from build123d import *

# Parameters (mm, degrees)
SKETCH1_R                        = 12.000000003
SKETCH1_R_2                      = 8.500000018
BOSS_EXTRUDE1_DEPTH              = 4.7625
SKETCH1_4_R                      = 9.525
CUT_EXTRUDE1_DEPTH               = 1.5875
F_10_32_TAPPED_HOLE1_D           = 4.0386
BOSS_EXTRUDE3_START              = -0.79375
SKETCH7_R                        = 8.500000018
SKETCH7_R_2                      = 6.5
BOSS_EXTRUDE3_DEPTH              = 0.79375
F_17_64_0_26563_DIAMETER_HOLE1_D = 6.747002
CUT_EXTRUDE2_DEPTH               = 0.7366


with BuildPart() as part:
    # Sketch1 → Boss-Extrude1 (new body)
    with BuildSketch(Plane.XY):
        with BuildLine():
            Line((-70.300649756, 35.543758941), (-22.715793489, -19.601472909))
            ThreePointArc((-22.715793489, -19.601472909), (6.372007721, -29.319320109), (28.80246523, -8.404939663))
            Line((28.80246523, -8.404939663), (49.20643424, 61.516396068))
            ThreePointArc((49.20643424, 61.516396068), (48.977980792, 61.993965606), (48.478121662, 61.819596767))
            ThreePointArc((48.478121662, 61.819596767), (47.697638407, 60.484610946), (46.853975269, 59.18862724))
            ThreePointArc((46.853975269, 59.18862724), (46.782773661, 59.083463588), (46.711157924, 58.978581516))
            ThreePointArc((46.711157924, 58.978581516), (13.35804262, 45.469068231), (-11.695774538, 71.300125033))
            ThreePointArc((-11.695774538, 71.300125033), (-16.142405131, 74.275551921), (-18.952954781, 69.722915382))
            ThreePointArc((-18.952954781, 69.722915382), (-31.025391021, 35.82315688), (-66.977119299, 34.270553581))
            ThreePointArc((-66.977119299, 34.270553581), (-67.0858071, 34.336250039), (-67.194235, 34.402374566))
            ThreePointArc((-67.194235, 34.402374566), (-68.499704148, 35.231284429), (-69.763880718, 36.121901549))
            ThreePointArc((-69.763880718, 36.121901549), (-70.291023197, 36.073070731), (-70.300649756, 35.543758941))
        make_face()
        Circle(SKETCH1_R, mode=Mode.SUBTRACT)
        with Locations((-7.832512348, 36.039494433)):
            Circle(SKETCH1_R_2, mode=Mode.SUBTRACT)
    extrude(amount=-BOSS_EXTRUDE1_DEPTH)

    # Sketch1_4 → Cut-Extrude1 (cut)
    with BuildSketch(Plane.XY):
        with Locations((-36.319050549, 15.602840887)):
            Circle(SKETCH1_4_R)
        with Locations((26.566795152, 29.269907275)):
            Circle(SKETCH1_4_R)
    extrude(amount=-CUT_EXTRUDE1_DEPTH, mode=Mode.SUBTRACT)

    # 10-32 Tapped Hole1 (through all)
    with Locations(Plane.XY):
        with Locations((-15.353270713, 70.644524994)):
            Hole(F_10_32_TAPPED_HOLE1_D / 2)

    # Sketch7 → Boss-Extrude3 (add)
    with BuildSketch(Plane(origin=(0, 0, -4.7625), x_dir=(-1, 0, 0), z_dir=(0, 0, -1)).offset(BOSS_EXTRUDE3_START)):
        with Locations(Location((7.832512348, 36.039494433, 0), (0, 0, 180))):
            Circle(SKETCH7_R)
        with Locations((7.832512348, 36.039494433)):
            Circle(SKETCH7_R_2, mode=Mode.SUBTRACT)
    extrude(amount=BOSS_EXTRUDE3_DEPTH)

    # 17_64 _0.26563_ Diameter Hole1 (through all)
    with Locations(Plane.XY):
        with Locations((-36.319050549, 15.602840887), (26.566795152, 29.269907275), (23.108788276, 10.542480941), (25.4, 0), (-23.108788276, -10.542480941), (-25.4, 0)):
            Hole(F_17_64_0_26563_DIAMETER_HOLE1_D / 2)

    # Sketch1_5 → Cut-Extrude2 (cut)
    with BuildSketch(Plane.XY):
        Polygon((-23.108641119, 3.96875), (-27.691358881, 3.96875), (-29.982717762, 0), (-27.691358881, -3.96875), (-23.108641119, -3.96875), (-20.817282238, 0), align=None)
        Polygon((-23.546192056, -15.104276642), (-19.376859203, -13.202181577), (-18.939455423, -8.640385876), (-22.671384497, -5.98068524), (-26.84071735, -7.882780306), (-27.27812113, -12.444576006), align=None)
        Polygon((23.546192056, 15.104276642), (19.376859203, 13.202181577), (18.939455423, 8.640385876), (22.671384497, 5.98068524), (26.84071735, 7.882780306), (27.27812113, 12.444576006), align=None)
        Polygon((27.691358881, 3.96875), (23.108641119, 3.96875), (20.817282238, 0), (23.108641119, -3.96875), (27.691358881, -3.96875), (29.982717762, 0), align=None)
    extrude(amount=-CUT_EXTRUDE2_DEPTH, mode=Mode.SUBTRACT)


solid = part.part
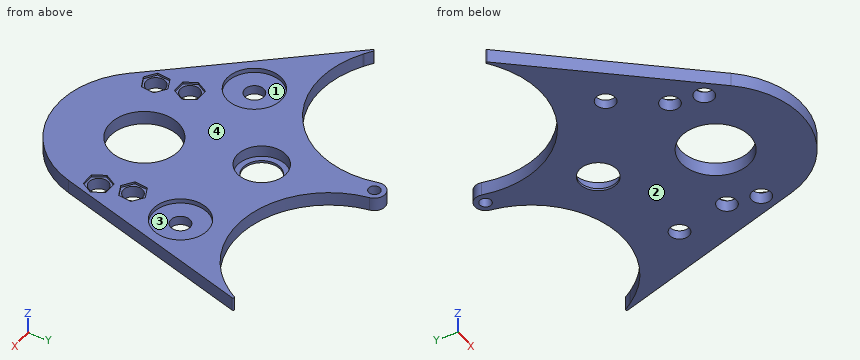
Build history of the part. All positions in model axes, mm. Face numbers are marked on the shaded views. A direction names the side the tool comes from. Round coordinates to 2 decimals unless told otherwise and drop trailing zeros. Write each loop counter-clockwise with the first axis right and the second up, starting at its lowest first coordinate (ties: lowest second). Pieces come first, ordered by that corner, then holes. Notation, with made-up numbers: M -17.5,-4.75 L 24.5,-4.75 A14 ccw 24.5,20.25 Z; hole C -2.75,-38.75 d2. An arc over 180 degrees is marked long. Answer as a JSON object with one key per item and string values. Group by question number.
(1) Drill centre lines: L1, parallel to Y at x = 0, z = -3.15; L2, parallel to Y at x = 25.4, z = -3.05; L3, parallel to Y at x = -1, z = -1.5. Where is each one in solid material? Low to high.
(2) Cut at A-A (x = -35.5). Give the cut face in (y, z).
(3) Flat gauge pins, fed straight in: pin 1 (0.8 mm diameter, centred on x = 25.5, z = -0.5, fed in from -Y); pin 2 (8 mm diameter, centred on x = 27.5, y = 27.5, fed in from +Z); pin 3 (1.5 mm diameter, centred on y = 9.5, z = -3.5, fed in from +X). Where does each tip first touch, or does it go through?
(4) Cut at B-B (y = 49.5). Give the cut face in (x, z).
(5) Which spindle directions (+Z, -Z, +X, -X, +Y, -Y) get a long thin tool onto all of the face, cutting with end or side? Do the marked faces 1 and 2. Say none if no direction does.
(6) Cut at D-D (y = -18). Give the cut face in (x, z).
(7) Mould opens along Y. For the marked faces 3 and 4 say: pulls with the +Y half, pulls with the -Y half, needs draft (parallel to the pull), parting line crosses it, or undercut.
(8) Cut at C-C (z = -2.85). Give the number of separate pieces and of enclosed holes in the cut face, and give its area (3 significant figures).
Responses:
{
 "1": {"L1": "y = -30 to -12, 12 to 32.74, 39.34 to 51.74", "L2": "y = -15.97 to -3.37, 3.37 to 8.07, 13.02 to 26.1, 32.44 to 45.23", "L3": "y = -29.99 to -11.96, 11.96 to 30.98, 41.1 to 52.57"},
 "2": {"outline": "M -4.79,-4.76 L 12.33,-4.76 L 12.33,-1.59 L 6.11,-1.59 L 6.11,0 L -4.79,0 Z; M 18.88,-4.76 L 33.05,-4.76 L 33.05,0 L 25.09,0 L 25.09,-1.59 L 18.88,-1.59 Z"},
 "3": {"pin 1": "stops at y = -16.44", "pin 2": "stops at z = -1.59", "pin 3": "stops at x = 34.25"},
 "4": {"outline": "M -20.36,-4.76 L 3.21,-4.76 L 3.21,0 L -20.36,0 Z; M 36.8,-4.76 L 45.7,-4.76 L 45.7,0 L 36.8,0 Z"},
 "5": {"face 1": "+Z", "face 2": "-Z, +X, -X, +Y, -Y"},
 "6": {"outline": "M -24.1,-4.76 L 24,-4.76 L 24,0 L -24.1,0 Z"},
 "7": {"face 3": "undercut", "face 4": "needs draft"},
 "8": {"separate pieces": "1", "enclosed holes": "9", "area": "4,850 mm2"}
}
